from build123d import *

# Parameters (mm, degrees)
BOSS_EXTRUDE1_DEPTH = 5
BOSS_EXTRUDE2_START = 5
SKETCH1_3_R         = 0.675
BOSS_EXTRUDE2_DEPTH = 2.5


with BuildPart() as part:
    # Sketch1 → Boss-Extrude1 (new body)
    with BuildSketch(Plane.XY):
        with BuildLine():
            ThreePointArc((4.5, 0), (-11.118671164, 40.613600031), (-54.5, 44))
            Line((-54.5, 44), (-54.5, 42))
            Line((-54.5, 42), (-39.5, 42))
            ThreePointArc((-39.5, 42), (-12.570901459, 28.857582118), (-4.5, 0))
            ThreePointArc((-4.5, 0), (0, -4.5), (4.5, 0))
        make_face()
        with BuildLine():
            Line((-2.900000039, 3.608329712), (-2.399984199, 15.608708951))
            ThreePointArc((-2.399984199, 15.608708951), (1e-09, 18), (2.399984199, 15.608708949))
            Line((2.399984199, 15.608708949), (2.899999961, 3.608329727))
            Line((2.899999961, 3.608329727), (2.899999994, 2.754995469))
            ThreePointArc((2.899999994, 2.754995469), (9e-09, -4), (-2.900000006, 2.754995456))
            Line((-2.900000006, 2.754995456), (-2.900000039, 3.608329712))
        make_face(mode=Mode.SUBTRACT)
    extrude(amount=BOSS_EXTRUDE1_DEPTH)

    # Sketch1<3> → Boss-Extrude2 (add)
    with BuildSketch(Plane.XY.offset(BOSS_EXTRUDE2_START)):
        with BuildLine():
            Line((2.899999967, 3.440930135), (2.899999961, 3.608329727))
            Line((2.899999961, 3.608329727), (2.399984199, 15.608708949))
            ThreePointArc((2.399984199, 15.608708949), (1e-09, 18), (-2.399984199, 15.608708951))
            Line((-2.399984199, 15.608708951), (-2.900000039, 3.608329712))
            Line((-2.900000039, 3.608329712), (-2.900000033, 3.440930079))
            ThreePointArc((-2.900000033, 3.440930079), (-1.84960355, 4.102312361), (-0.658476506, 4.4515625))
            ThreePointArc((-0.658476506, 4.4515625), (0, 5.275), (0.658476506, 4.4515625))
            ThreePointArc((0.658476506, 4.4515625), (1.849603511, 4.102312379), (2.899999967, 3.440930135))
        make_face()
        with Locations((0, 11.2)):
            Circle(SKETCH1_3_R, mode=Mode.SUBTRACT)
        with Locations((0, 13.4)):
            Circle(SKETCH1_3_R, mode=Mode.SUBTRACT)
        with Locations((0, 15.6)):
            Circle(SKETCH1_3_R, mode=Mode.SUBTRACT)
        with Locations((0, 6.8)):
            Circle(SKETCH1_3_R, mode=Mode.SUBTRACT)
        with Locations((0, 9)):
            Circle(SKETCH1_3_R, mode=Mode.SUBTRACT)
    extrude(amount=-BOSS_EXTRUDE2_DEPTH)


solid = part.part
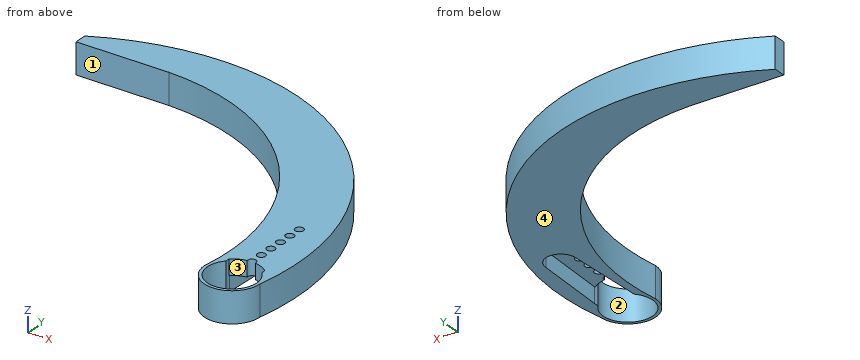
Could you check a few things on this model? Use its own coordinates, in mm. Face numbers are marked on the shaded views. Round coordinates to 2 decimals unless told otherwise and drop trailing zeros. Order: outer loops, then holes, each group sorted by start corner. A loop starts at its lowest first (then second) coordinate and runs counter-clockwise, first axis right, second up.
Q1. Please list where these lines run through material, in increasing order: probe 1 along X at (y, z) = (6, 1.85); probe 2 along X at (y, z) = (-2, 3.3); probe 3 along Z at (x, y) = (-1.5, 12).
Geometry says:
probe 1: x = -4.1 to -2.8, 2.8 to 5.23
probe 2: x = -4.03 to -3.46, 3.46 to 4.03
probe 3: z = 2.5 to 5
Q2. Thinking about a two-plate mould opening in Y: for the marked faces 1, 2, 3 and 4, which applies, released by +Y, released by -Y, zero draft, split by the parting line, or undercut?
Geometry says:
face 1: released by -Y
face 2: undercut
face 3: undercut
face 4: zero draft
Q3. Imagine slicing it at D-D, the plane y = 13.4. List the corners of the cut face in (x, z) for me (3 decimals), then the cut area to 3 significant figures.
Geometry says:
outline: (-4.969, 0) - (-2.492, 0) - (-2.492, 2.5) - (-0.675, 2.5) - (-0.675, 5) - (-4.969, 5) - close; (0.675, 2.5) - (2.492, 2.5) - (2.492, 0) - (4.91, 0) - (4.91, 5) - (0.675, 5) - close
area: 33.6 mm2
Q4. Imagine slicing it at A-A, the plane y = 6.8. List the corners of the cut face in (x, z) for me (3 decimals).
Geometry says:
outline: (-4.118, 0) - (-2.767, 0) - (-2.767, 2.5) - (-0.675, 2.5) - (-0.675, 5) - (-4.118, 5) - close; (0.675, 2.5) - (2.767, 2.5) - (2.767, 0) - (5.263, 0) - (5.263, 5) - (0.675, 5) - close
Q5. I'm going to push flat-ended pins straight in: P1, Ø1.8, axis at x = 0, y = 6.8, coming from the -Z side; P2, Ø3, axis at y = 10, z = 3, coming from the +X side; P3, Ø2, axis at y = 22.5, z = 3.5, coming from the -X side. Where does each tip first touch, or does it pass through?
Geometry says:
P1: stops at z = 2.5
P2: stops at x = 5.27
P3: stops at x = -8.86
Q6. Imagine slicing it at B-B, the plane z = 1.55. List the corners of the cut face in (x, y) for me (1 decimal).
Geometry says:
outline: (-54.5, 42) - (-39.5, 42) arc R36.6 cw to (-4.5, 0) arc R4.5 ccw to (4.5, 0) arc R40.8 ccw to (-54.5, 44) - close; hole (-2.9, 2.8) arc R4 ccw (long way) to (2.9, 2.8) - (2.9, 3.6) - (2.4, 15.6) arc R2.4 ccw to (-2.4, 15.6) - (-2.9, 3.6) - close
Q7. Imagine slicing it at C-C, the plane x = 0. State how many separate pieces and enclosed holes the cut face has, then the cut area to 3 significant figures.
Geometry says:
separate pieces: 7
enclosed holes: 0
area: 67.4 mm2
